```python
from build123d import *

# Parameters (mm, degrees)
BOSS_EXTRUDE1_DEPTH = 6.35
CUT_EXTRUDE1_DEPTH  = 7.35
SKETCH3_W           = 6.35
SKETCH3_H           = 6.35
CUT_EXTRUDE2_DEPTH  = 7.35
SKETCH4_W           = 12.7
SKETCH4_H           = 6.35
SKETCH4_W_2         = 6.35
CUT_EXTRUDE3_DEPTH  = 7.35


with BuildPart() as part:
    # Sketch1 → Boss-Extrude1 (new body)
    with BuildSketch(Plane(origin=(0, 0, 0), x_dir=(1, 0, 0), z_dir=(0, 1, 0))):
        Polygon((-45.492088676, -38.013071454), (-45.492088676, 94.616309142), (110.168142166, 225.23075143), (110.168142166, 92.601370834), align=None)
    extrude(amount=BOSS_EXTRUDE1_DEPTH)

    # Sketch2 → Cut-Extrude1 (cut, through all)
    with BuildSketch(Plane(origin=(0, 6.35, 0), x_dir=(1, 0, 0), z_dir=(0, 1, 0))):
        Polygon((-45.492088676, -38.013071454), (-16.305795393, -13.522863525), (-20.387496714, -8.658481312), (-49.573789997, -33.148689241), align=None)
        Polygon((-0.929967859, 7.668323974), (3.151733462, 2.803941761), (22.609262318, 19.130747047), (18.527560996, 23.995129261), align=None)
        Polygon((37.985089851, 40.321934547), (42.066791173, 35.457552333), (61.524320028, 51.784357619), (57.442618706, 56.648739833), align=None)
        Polygon((80.981848883, 68.111162905), (115.03252438, 96.683072155), (110.950823058, 101.547454369), (76.900147562, 72.975545119), align=None)
    extrude(amount=-CUT_EXTRUDE1_DEPTH, mode=Mode.SUBTRACT)

    # Sketch3 → Cut-Extrude2 (cut, through all)
    with BuildSketch(Plane(origin=(0, 6.35, 0), x_dir=(1, 0, 0), z_dir=(0, 1, 0))):
        with Locations((106.993142166, 135.815707121)):
            Rectangle(SKETCH3_W, SKETCH3_H)
        with Locations((106.993142166, 123.115707121)):
            Rectangle(SKETCH3_W, SKETCH3_H)
        with Locations((106.993142166, 110.415707121)):
            Rectangle(SKETCH3_W, SKETCH3_H)
        with Locations((106.993142166, 148.515707121)):
            Rectangle(SKETCH3_W, SKETCH3_H)
        with Locations((106.993142166, 173.915707121)):
            Rectangle(SKETCH3_W, SKETCH3_H)
        with Locations((106.993142166, 186.615707121)):
            Rectangle(SKETCH3_W, SKETCH3_H)
        with Locations((106.993142166, 212.015707121)):
            Rectangle(SKETCH3_W, SKETCH3_H)
        with Locations((106.993142166, 161.215707121)):
            Rectangle(SKETCH3_W, SKETCH3_H)
        with Locations((106.993142166, 199.315707121)):
            Rectangle(SKETCH3_W, SKETCH3_H)
    extrude(amount=-CUT_EXTRUDE2_DEPTH, mode=Mode.SUBTRACT)

    # Sketch4 → Cut-Extrude3 (cut, through all)
    with BuildSketch(Plane(origin=(0, 6.35, 0), x_dir=(1, 0, 0), z_dir=(0, 1, 0))):
        with Locations((-39.142088676, -26.548735167)):
            Rectangle(SKETCH4_W, SKETCH4_H)
        with Locations((-42.317088676, -1.148735167)):
            Rectangle(SKETCH4_W_2, SKETCH4_H)
        with Locations((-42.317088676, -13.848735167)):
            Rectangle(SKETCH4_W_2, SKETCH4_H)
        with Locations((-42.317088676, 11.551264833)):
            Rectangle(SKETCH4_W_2, SKETCH4_H)
        with Locations((-42.317088676, 24.251264833)):
            Rectangle(SKETCH4_W_2, SKETCH4_H)
        with Locations((-42.317088676, 36.951264833)):
            Rectangle(SKETCH4_W_2, SKETCH4_H)
        with Locations((-42.317088676, 49.651264833)):
            Rectangle(SKETCH4_W_2, SKETCH4_H)
        with Locations((-42.317088676, 62.351264833)):
            Rectangle(SKETCH4_W_2, SKETCH4_H)
        with Locations((-42.317088676, 75.051264833)):
            Rectangle(SKETCH4_W_2, SKETCH4_H)
        with Locations((-42.317088676, 87.751264833)):
            Rectangle(SKETCH4_W_2, SKETCH4_H)
        with Locations((-42.317088676, 100.451264833)):
            Rectangle(SKETCH4_W_2, SKETCH4_H)
    extrude(amount=-CUT_EXTRUDE3_DEPTH, mode=Mode.SUBTRACT)


solid = part.part
```
Here's how the part is built. I have some questions about the finished solid (model axes, mm). A direction names the side the tool comes from. Coordinates: 2 decimals unless noted, no trailing zeros. Loops run counter-clockwise (first coordinate to the right, second up) from the corner with the lowest first, then second, coordinate; pieces in that order, holes last. Notation, with made-up numbers: (2, -23.75) -> (52, -23.75) arc R28 cw to (52, 11.25) -> close; hole circle Ø1 at (-0.5, 4.25). An arc over 180 degrees is marked (long way). Return JSON: item names as keys, results as strings.
1) Thinking about a two-plate mould opening in X: for faces 1 (the face through (78.91, 3.22, -70.58)), 2 (the face through (-45.492, 3, -43)), 3 (the face through (-42, 3, -78.226)), 4 (the face through (-18.32, 3.22, 11.12)), which applies, +X half, -X half, draft (parallel to the pull), parting line (faces both ways), or undercut?
Results below:
{"face 1": "+X half", "face 2": "-X half", "face 3": "draft", "face 4": "undercut"}
2) I need wall thicknesses on line 1 (Z direction, x = 78.5, y = 3.75); line 2 (Z direction, x = 22.5, y = 3.25); line 3 (X direction, y = 1.25, z = -38). Which ranges of each line are inside material? Lowest first, please. Write a range as from..to.
Results below:
{"line 1": "-198.66..-74.32, -71.07..-66.03", "line 2": "-151.67..-19.26", "line 3": "-39.14..39.93"}
3) If we section it at A-A, the plane x = -34: Write out the boundary of the cut face in (y, z), then the cut area to 3 significant figures.
Results below:
{"outline": "(0, -104.26) -> (6.35, -104.26) -> (6.35, 20.08) -> (0, 20.08) -> close", "area": "790 mm²"}
4) Will these pins go through, and if not, where does the flat tip stop? pin 1 (3 mm diameter, centred on x = 107, y = 2.5, fed in from +Z); pin 2 (3 mm diameter, centred on y = 2.5, z = -86.5, fed in from -X); pin 3 (2 mm diameter, centred on x = 72, y = 1, fed in from -Z).
Results below:
{"pin 1": "z = -96.97", "pin 2": "x = -39.14", "pin 3": "z = -194.04"}
5) For faces 5 (the face through (9, 3, -16)), 6 (the face through (-42, 3, 23.374)), 7 (the face through (-42, 3, -2.026)), 8 (the face through (103.818, 3, -161)), which set-ups out of +Z, -Z, +X, -X, +Y, -Y let a thin tool reach every point of the face, with its end or its side?
Results below:
{"face 5": "+Y, -Y", "face 6": "+Z, +X, -X, +Y, -Y", "face 7": "-X, +Y, -Y", "face 8": "+X, +Y, -Y"}
6) If we section it at B-B, the plane z = -130: Write out the boundary of the cut face in (x, y), then the cut area to 3 significant figures.
Results below:
{"outline": "(-3.32, 0) -> (110.17, 0) -> (110.17, 6.35) -> (-3.32, 6.35) -> close", "area": "721 mm²"}
